Read the model definition and answer for the solid it produces. Units are mm, in the model's axes. Face numbers are marked on the shaded views. A direction names the side the tool comes from. Give positions to 0.01 mm unless a question says otherwise; leave off trailing zeros. Order: outer loops, then holes, each group sorted by start corner. A loop starts at its lowest first (then second) coordinate and runs counter-clockwise, first axis right, second up. Notation, with made-up numbers: (-18.75, 55) - (-6.75, 55) arc R11 cw to (-6.75, 74) - close; hole circle Ø3 at (89.25, 57.5). An arc over 180 degrees is marked (long way). Return JSON: item names as keys, results as strings.
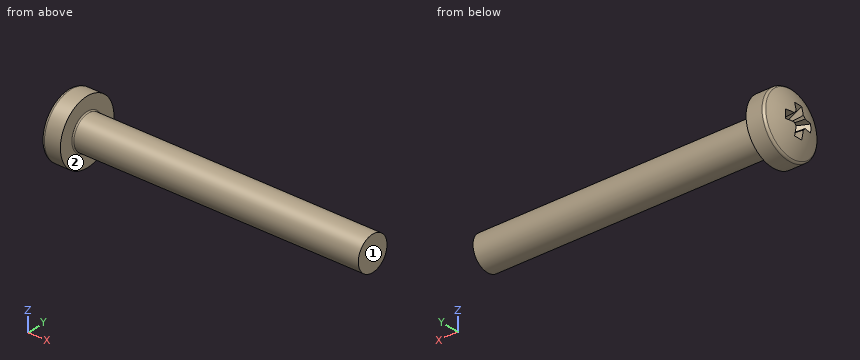
```python
from build123d import *

# Parameters (mm, degrees)
FILLET1_R    = 0.1
RECPAT_COUNT = 2
RECPAT_ANGLE = 90


with BuildPart() as part:
    # BodySke → Base-Revolve (revolve)
    with BuildSketch(Plane.XY, mode=Mode.PRIVATE) as base_revolve_sk:
        with BuildLine():
            Line((2.4, 1.5), (2.4, 2.8))
            Line((2.4, 2.8), (1.003501533, 2.8))
            ThreePointArc((1.003501533, 2.8), (0.873295971, 2.76653015), (0.775371599, 2.674418605))
            ThreePointArc((0.775371599, 2.674418605), (0.197753546, 1.392274756), (0, 0))
            Line((0, 0), (27.4, 0))
            Line((27.4, 0), (27.4, 1.5))
            Line((27.4, 1.5), (2.4, 1.5))
        make_face()
    revolve(base_revolve_sk.sketch.rotate(Axis((1.003501533, 0, 0), (1, 0, 0)), 90), axis=Axis((1.003501533, 0, 0), (1, 0, 0)))

    # Fillet1
    fillet1_edges = [part.edges().sort_by_distance(p)[0] for p in [
        (2.4, 0, -1.5),
    ]]
    fillet(fillet1_edges, radius=FILLET1_R)

    # Sketch3 → Recess section 0
    with BuildSketch(Plane(origin=(0, 0, 0), x_dir=(0, 0, -1), z_dir=(1, 0, 0))):
        with BuildLine():
            Line((0.37, -1.4), (-0.37, -1.4))
            Line((-0.37, -1.4), (-0.37, 1.4))
            Line((-0.37, 1.4), (0.37, 1.4))
            Line((0.37, 1.4), (0.37, -1.4))
        make_face()
    # Sketch4 → Recess section 1
    with BuildSketch(Plane(origin=(1.75, 0, 0), x_dir=(0, 0, -1), z_dir=(1, 0, 0))):
        with BuildLine():
            Line((0.37, -0.527482332), (-0.37, -0.527482332))
            Line((-0.37, -0.527482332), (-0.37, 0.527482332))
            Line((-0.37, 0.527482332), (0.37, 0.527482332))
            Line((0.37, 0.527482332), (0.37, -0.527482332))
        make_face()
    recess = loft(mode=Mode.SUBTRACT)

    # RecPat: Recess ×2 about axis
    recpat_axis = Axis((0, 0, 0), (1, 0, 0))
    for i in range(1, RECPAT_COUNT):
        add(recess.rotate(recpat_axis, i * RECPAT_ANGLE / (RECPAT_COUNT - 1)), mode=Mode.SUBTRACT)

    # RecCorSke → RecessCore (revolve, cut)
    with BuildSketch(Plane.XY, mode=Mode.PRIVATE) as recesscore_sk:
        Polygon((0, 0), (0, 0.678371921), (1.75, 0.556), (1.930655351, 0), align=None)
    revolve(recesscore_sk.sketch.rotate(Axis((-3.175, 0, 0), (1, 0, 0)), 15.814025638), axis=Axis((-3.175, 0, 0), (1, 0, 0)), mode=Mode.SUBTRACT)


solid = part.part
```
Q1. Consider L1, parallel to X at y = 0.1, z = 2; L2, parallel to Z at x = 10.75, y = -0.75; L3, parallel to Y at x = 9.5, z = -0.85. Determine where each line is inside the solid, lowest interval first.
Values:
{"L1": "x = 0.42 to 2.4", "L2": "z = -1.3 to 1.3", "L3": "y = -1.24 to 1.24"}
Q2. For the marked faces 1 and 2, determine the directions among +Z, -Z, +X, -X, +Y, -Y from which every point of the face is accessible in a straight line to the end or side of a thin tool.
Values:
{"face 1": "+Z, -Z, +X, +Y, -Y", "face 2": "+X"}
Q3. Given pin 1 (1.5 mm diameter, centred on x = 20.5, z = 0, fed in from -Y), flat-ended and moving along its own axis, determine where the tip first touches the part or whether it passes through.
Values:
{"pin 1": "stops at y = -1.5"}
Q4. A cutting plane is placed at A-A (x = 18). Write down the section's boundary in (y, z).
Values:
{"outline": "circle Ø3 at (0, 0)"}
